CAD build for the part. Positions are in the model's coordinates, mm. A direction names the side the tool comes from. Give positions to 0.01 mm unless a question says otherwise; leave off trailing zeros.
```python
from build123d import *


with BuildPart() as part:
    # Balayage1: sweep along a path in Esquisse1
    with BuildLine(Plane.XY) as balayage1_path:
        Line((48.792061638, 17.109637903), (6.141771071, 45.25804309))
        ThreePointArc((6.141771071, 45.25804309), (0, 47.102069304), (-6.141771071, 45.25804309))
        Line((-6.141771071, 45.25804309), (-48.792061638, 17.109637903))
        ThreePointArc((-48.792061638, 17.109637903), (-57.134139235, -5.895015818), (-37.50001617, -20.5))
        Line((-37.50001617, -20.5), (37.50001617, -20.5))
        ThreePointArc((37.50001617, -20.5), (57.134139235, -5.895015818), (48.792061638, 17.109637903))
    # Esquisse2 → Balayage1 (sweep)
    with BuildSketch(Plane(origin=(0, 0, 0), x_dir=(0, 0, -1), z_dir=(1, 0, 0))):
        with BuildLine():
            Line((-4.5, -20.5), (-2.5, -20.5))
            Line((-2.5, -20.5), (-2.5, -26.5))
            Line((-2.5, -26.5), (2.5, -26.5))
            Line((2.5, -26.5), (2.5, -20.5))
            Line((2.5, -20.5), (4.5, -20.5))
            Line((4.5, -20.5), (6, -24.208099244))
            ThreePointArc((6, -24.208099244), (6.228715258, -26.416259945), (5.244821685, -28.406294565))
            Line((5.244821685, -28.406294565), (3.458805812, -30.360920906))
            ThreePointArc((3.458805812, -30.360920906), (2.286874079, -31.202594508), (0.875, -31.5))
            Line((0.875, -31.5), (-0.875, -31.5))
            ThreePointArc((-0.875, -31.5), (-2.286874079, -31.202594508), (-3.458805812, -30.360920906))
            Line((-3.458805812, -30.360920906), (-5.244821685, -28.406294565))
            ThreePointArc((-5.244821685, -28.406294565), (-6.228715258, -26.416259945), (-6, -24.208099244))
            Line((-6, -24.208099244), (-4.5, -20.5))
        make_face()
    sweep(path=balayage1_path.line)


solid = part.part
```
1. Probe line 1 along Z through (x, y) = (53, -16); line 2 along X through (y, z) = (43, -4.25); line 3 along Y through (x, z) = (32.5, -2.75). List the from-to ranges inside material, lowest first.
Responses:
line 1: z = -5.22 to -2.5, 2.5 to 5.22
line 2: x = -25.89 to -9.56, 9.56 to 25.89
line 3: y = -30.96 to -20.5, 27.86 to 40.39
2. Drop flat-ended pins along their axis: pin 1 (2 mm diameter, centred on x = 16.5, z = 3.5, fed in from +Y); pin 2 (1.5 mm diameter, centred on y = 38, z = 0.5, fed in from +X); pin 3 (0.6 mm diameter, centred on x = -0.5, z = -3.5, fed in from +Y). Give the stop position or say it passes through.
Responses:
pin 1: stops at y = 51.39
pin 2: stops at x = 38.25
pin 3: stops at y = 57.21
3. Tool access for faces 1 (the face through (-27.765, 30.987, 3.486)), 2 (the face through (-63.013, -7.165, 0.035)), 3 (the face through (0.525, -31.194, 2.305)), 4 (the face through (57.246, -6.316, 4.594)), 5 (the face through (-57.41, -5.591, -4.573)): list every direction of +Z, -Z, +X, -X, +Y, -Y with a clear straight run to the whole face (end or side of a thin tool).
Responses:
face 1: +Z, -Z
face 2: none
face 3: +Z, +X, -X, -Y
face 4: +Z
face 5: -Z
4. Pull direction X, two halves, no side cores. Call faces 6 (the face through (28.18, 32.91, 5.24)), 7 (the face through (-65.15, -7.76, -4.96)), 8 (the face through (32.069, 38.807, -4.339)): released by +X, released by -X, zero draft, split by the parting line, or undercut.
Responses:
face 6: undercut
face 7: released by -X
face 8: released by +X
